Build history of the part. All positions in model axes, mm. A direction names the side the tool comes from. Coordinates: 2 decimals unless noted, no trailing zeros. Loops run counter-clockwise (first coordinate to the right, second up) from the corner with the lowest first, then second, coordinate; pieces in that order, holes last. Notation, with made-up numbers: (52, 50) -> (78, 50) arc R5 ccw to (78, 55) -> close; hole circle Ø1 at (89, 33). An arc over 180 degrees is marked (long way). One line per item, written item: value. Start each with the question number.
```python
from build123d import *

# Parameters (mm, degrees)
SKETCH_W     = 30
SKETCH_H     = 20
PAD_DEPTH    = 2
SKETCH001_W  = 9.5
SKETCH001_H  = 1.3
PAD001_DEPTH = 10
SKETCH002_W  = 9.5
SKETCH002_H  = 2.2
PAD002_DEPTH = 1.3


with BuildPart() as part:
    # Sketch → Pad (new body)
    with BuildSketch(Plane.XY):
        Rectangle(SKETCH_W, SKETCH_H)
    extrude(amount=PAD_DEPTH)

    # Sketch001 (on Face6 of Pad) → Pad001 (join)
    with BuildSketch(Plane.XY.offset(2)):
        with Locations((0, 9.35)):
            Rectangle(SKETCH001_W, SKETCH001_H)
        with Locations((0, -9.35)):
            Rectangle(SKETCH001_W, SKETCH001_H)
    extrude(amount=PAD001_DEPTH)

    # Sketch002 (on Face16 of Pad001) → Pad002 (join)
    with BuildSketch(Plane.XY.offset(12)):
        with Locations((0, 8.9)):
            Rectangle(SKETCH002_W, SKETCH002_H)
    extrude(amount=-PAD002_DEPTH)


solid = part.part
```
Item 1: Band-saw the part on A-A, the plane z = 6. List the corners of the cut face in (x, y), and give its area (3 significant figures).
Item 2: Drop flat-ended pins along their axis: pin 1 Ø0.7 at (y, z) = (8.5, 8) entering from -X; pin 2 Ø5 at (x, z) = (6.5, 8) entering from +Y; pin 3 Ø1 at (x, y) = (12, -6.5) entering from +Z; pin 4 Ø1.1 at (y, z) = (9.5, 5.5) entering from +X. Give the stop position or say it passes through.
Item 3: Tool access for faces 1 (the face through (0, -8.7, 7)), 2 (the face through (4.75, 9, 7)), 3 (the face through (-4.75, 9, 7)): list every direction of +Z, -Z, +X, -X, +Y, -Y with a clear straight run to the whole face (end or side of a thin tool).
Item 4: Band-saw the part on D-D, the plane x = 7. List the corners of the cut face in (y, z), and give its area (3 significant figures).
Item 5: Probe probe 1 along Y at (x, z) = (1.75, 6.25); probe 2 along Z at (x, y) = (11.5, -1.25); probe 3 along X at (y, z) = (-9, 2.5). List the from-to ranges inside material, lowest first.
Item 6: Two-plate mould, pull along Z, no slides. Class faces 4 (the face through (4.75, -9, 7)), 5 (the face through (0, 9, 12)), 6 (the face through (0, 8.7, 6)), 7 (the face through (0, 8, 10.7)): +Z half, -Z half, draft (parallel to the pull), parting line (faces both ways), or undercut.
Item 7: Band-saw the part on B-B, the plane x = -0.75. List the corners of the cut face in (y, z), and give its area (3 significant figures).
Item 8: Band-saw the part on C-C, the plane y = 0. List the corners of the cut face in (x, z), and give its area (3 significant figures).
Worked out:
1. outline: (-4.75, -10) -> (4.75, -10) -> (4.75, -8.7) -> (-4.75, -8.7) -> close; (-4.75, 8.7) -> (4.75, 8.7) -> (4.75, 10) -> (-4.75, 10) -> close
1. area: 24.7 mm²
2. pin 1: stops at x = -4.75
2. pin 2: stops at y = 10
2. pin 3: stops at z = 2
2. pin 4: stops at x = 4.75
3. face 1: +Z, +X, -X
3. face 2: +Z, +X, +Y, -Y
3. face 3: +Z, -X, +Y, -Y
4. outline: (-10, 0) -> (10, 0) -> (10, 2) -> (-10, 2) -> close
4. area: 40.0 mm²
5. probe 1: y = -10 to -8.7, 8.7 to 10
5. probe 2: z = 0 to 2
5. probe 3: x = -4.75 to 4.75
6. face 4: draft
6. face 5: +Z half
6. face 6: undercut
6. face 7: undercut
7. outline: (-10, 0) -> (10, 0) -> (10, 12) -> (7.8, 12) -> (7.8, 10.7) -> (8.7, 10.7) -> (8.7, 2) -> (-8.7, 2) -> (-8.7, 12) -> (-10, 12) -> close
7. area: 67.2 mm²
8. outline: (-15, 0) -> (15, 0) -> (15, 2) -> (-15, 2) -> close
8. area: 60.0 mm²
